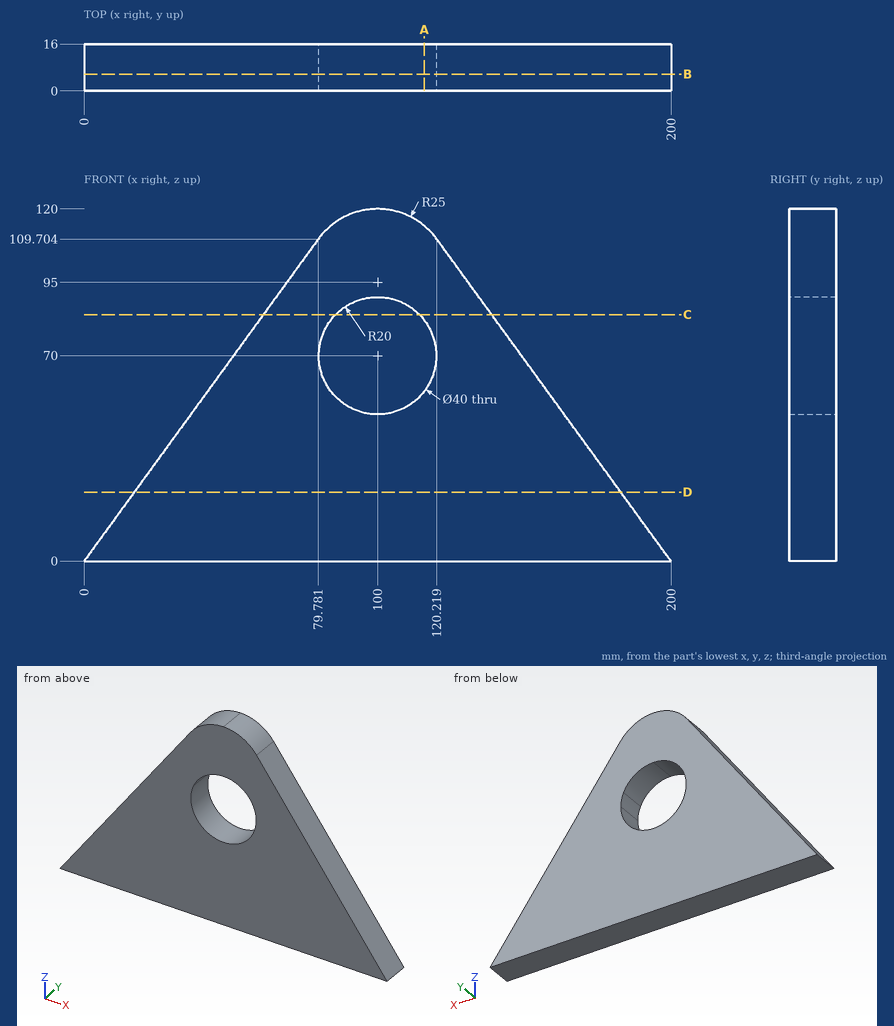
Can you work these out from the drawing? Everything is in mm from the part's minimum corner. Coordinates: 2 decimals unless noted, no trailing zeros. Loops run counter-clockwise (first coordinate to the right, second up) from the corner with the lowest first, then second, coordinate; pieces in that order, holes last. Notation, with made-up numbers: (-1, 79) -> (38, 79) arc R22 cw to (38, 100) -> close; hole circle Ø8 at (75.5, 51). An arc over 180 degrees is marked (long way). Return JSON: item names as keys, results as strings.
1) If we section it at B-B, the plane y = 5.75: Write out the boundary of the cut face in (x, z).
Results below:
{"outline": "(0, 0) -> (200, 0) -> (120.22, 109.7) arc R25 ccw to (100, 120) arc R25 ccw to (79.78, 109.7) -> close; hole (81.67, 78) arc R20 ccw (long way) to (120, 70) arc R20 ccw to (118.33, 78) arc R20 ccw to (100, 90) arc R20 ccw to start"}
2) Will these pins go through, and if not, where does the flat tip stop? pin 1 (4 mm diameter, centred on y = 12, z = 32.5, fed in from -X); pin 2 (1 mm diameter, centred on y = 9.5, z = 94, fed in from -X); pin 3 (8 mm diameter, centred on x = 58, z = 91.5, fed in from +Y); pin 4 (1.5 mm diameter, centred on x = 76, y = 9.5, fed in from +Z) (1 decimal).
Results below:
{"pin 1": "x = 22.18", "pin 2": "x = 68", "pin 3": "through", "pin 4": "z = 105.5"}
3) If we section it at D-D, the plane z = 23.5: Write out the boundary of the cut face in (x, y).
Results below:
{"outline": "(17.09, 0) -> (182.91, 0) -> (182.91, 16) -> (17.09, 16) -> close"}
4) If we section it at A-A, the plane x = 116: Write out the boundary of the cut face in (y, z), then the cut area to 3 significant figures.
Results below:
{"outline": "(0, 0) -> (16, 0) -> (16, 58) -> (0, 58) -> close; (0, 82) -> (16, 82) -> (16, 114.21) -> (0, 114.21) -> close", "area": "1,440 mm²"}
5) I need wall thicknesses on line 1 (Z direction, x = 100, y = 3.75); line 2 (X direction, y = 5, z = 55.5) (1 decimal); line 3 (X direction, y = 8.25, z = 70.5) (1 decimal). Which ranges of each line are inside material? Lowest first, please. Write a range as from..to.
Results below:
{"line 1": "0..50, 90..120", "line 2": "40.4..86.2, 113.8..159.6", "line 3": "51.3..80, 120..148.7"}
6) If we section it at C-C, the plane z = 84: Write out the boundary of the cut face in (x, y).
Results below:
{"outline": "(61.09, 0) -> (85.72, 0) -> (85.72, 16) -> (61.09, 16) -> close; (114.28, 0) -> (138.91, 0) -> (138.91, 16) -> (114.28, 16) -> close"}
